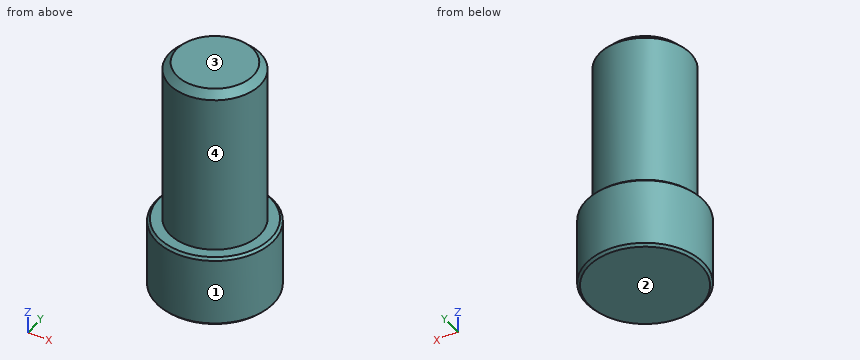
from build123d import *

# Parameters (mm, degrees)
F0_R     = 1.9
F1_DEPTH = 10
F0_R_2   = 2.45
F2_DEPTH = 3
F3_SIZE  = 0.3
F4_SIZE  = 0.1


with BuildPart() as f1:
    # F0 (on Top) → F1 (new body)
    with BuildSketch(Plane.XY):
        Circle(F0_R)
    extrude(amount=F1_DEPTH)

    # F0 (on Top) → F2 (join)
    with BuildSketch(Plane.XY):
        Circle(F0_R_2)
        Circle(F0_R, mode=Mode.SUBTRACT)
    extrude(amount=F2_DEPTH)

    # F3
    f3_edges = [f1.edges().sort_by_distance(p)[0] for p in [
        (-1.9, 0, 10),
    ]]
    chamfer(f3_edges, length=F3_SIZE)

    # F4
    f4_edges = [f1.edges().sort_by_distance(p)[0] for p in [
        (-2.45, 0, 0),
        (-2.45, 0, 3),
    ]]
    chamfer(f4_edges, length=F4_SIZE)


solid = f1.part
Work out the finished part from the listing and answer in its coordinate system (mm). Face numbers are marked on the shaded views. A direction names the side the tool comes from. Round coordinates to 2 decimals unless told otherwise and drop trailing zeros. Write each loop counter-clockwise with the first axis right and the second up, starting at its lowest first coordinate (ties: lowest second). Pieces come first, ordered by that corner, then holes.
1) A tool of negligible diameter and unlimited length cuts with its end or side. For the marked faces 3 and 4, from which of +Z, -Z, +X, -X, +Y, -Y can it reach the whole face along a straight path? Write none if from no direction.
2) The mould has two halves that part along Y. Classify the marked faces 1 and 2: pulls with the +Y half, pulls with the -Y half, needs draft (parallel to the pull), parting line crosses it, or undercut.
3) A cutting plane is placed at D-D (z = 1.5). Give the vertices of the cut face in (x, y).
4) A cutting plane is placed at A-A (y = 0). Give the vertices of the cut face in (x, z), plus the area to 3 significant figures.
5) Straight lines are drawn through the part: line 1 (Z direction, x = 0.7, y = 2.2); line 2 (Y direction, x = 0.1, z = 0.5); line 3 (X direction, y = 1, z = 0.75). For each, find the intervals that lie inside material, in ascending order.
6) A cutting plane is placed at C-C (z = 7.25). Give the vertices of the cut face in (x, y), plus the area to 3 significant figures.
Completed:
1. face 3: +Z, +X, -X, +Y, -Y
1. face 4: +Z
2. face 1: parting line crosses it
2. face 2: needs draft
3. outline: circle Ø4.9 at (0, 0)
4. outline: (-2.45, 0.1) - (-2.35, 0) - (2.35, 0) - (2.45, 0.1) - (2.45, 2.9) - (2.35, 3) - (1.9, 3) - (1.9, 9.7) - (1.6, 10) - (-1.6, 10) - (-1.9, 9.7) - (-1.9, 3) - (-2.35, 3) - (-2.45, 2.9) - close
4. area: 41.2 mm2
5. line 1: z = 0 to 3
5. line 2: y = -2.45 to 2.45
5. line 3: x = -2.24 to 2.24
6. outline: circle Ø3.8 at (0, 0)
6. area: 11.3 mm2
